from build123d import *

# Parameters (mm, degrees)
SKETCH063_W          = 88
SKETCH063_H          = 3
PAD030_DEPTH         = 176
SKETCH064_R          = 25
POCKET030_DEPTH      = 100
POCKET030_DEPTH_BACK = 100
PAD031_DEPTH         = 19
SKETCH066_W          = 139
SKETCH066_H          = 6
SKETCH066_W_2        = 6
SKETCH066_H_2        = 69.5
POCKET031_DEPTH      = 20
SKETCH067_W          = 3
SKETCH067_H          = 88
PAD032_DEPTH         = 19
SKETCH068_W          = 3
SKETCH068_H          = 79
PAD033_DEPTH         = 6
PAD033_DEPTH_BACK    = 6
CHAMFER009_SIZE      = 2.99
CHAMFER010_SIZE      = 1.5
FILLET017_R          = 2.99
SKETCH087_W          = 67
SKETCH087_H          = 4.5
PAD038_DEPTH         = 3
CHAMFER012_SIZE      = 2.99
CHAMFER014_SIZE      = 1


with BuildPart() as part:
    # Sketch063 → Pad030 (new body)
    with BuildSketch(Plane.YZ):
        with Locations((-44, 20.5)):
            Rectangle(SKETCH063_W, SKETCH063_H)
    extrude(amount=PAD030_DEPTH)

    # Sketch064 → Pocket030 (cut, two sides)
    with BuildSketch(Plane.XY) as pocket030_sk:
        with Locations((45.5, -45.5)):
            Circle(SKETCH064_R)
        with Locations((130.5, -45.5)):
            Circle(SKETCH064_R)
    extrude(amount=-POCKET030_DEPTH, mode=Mode.SUBTRACT)
    extrude(pocket030_sk.sketch, amount=POCKET030_DEPTH_BACK, mode=Mode.SUBTRACT)

    # Sketch065 → Pad031 (join)
    with BuildSketch(Plane.XY):
        with BuildLine():
            ThreePointArc((0, -12.5), (8.838835, -8.838835), (12.5, 0))
            Line((0, 0), (12.5, 0))
            Line((0, -12.5), (0, 0))
        make_face()
        with BuildLine():
            ThreePointArc((163.5, 0), (169.75, -6.25), (176, 0))
            Line((163.5, 0), (176, 0))
        make_face()
        with BuildLine():
            ThreePointArc((94.25, -88), (88, -81.75), (81.75, -88))
            Line((81.75, -88), (94.25, -88))
        make_face()
    extrude(amount=PAD031_DEPTH)

    # Sketch066 → Pocket031 (cut)
    with BuildSketch(Plane.XY):
        with Locations((88, -3)):
            Rectangle(SKETCH066_W, SKETCH066_H)
        with Locations((3, -53.25)):
            Rectangle(SKETCH066_W_2, SKETCH066_H_2)
    extrude(amount=POCKET031_DEPTH, mode=Mode.SUBTRACT)

    # Sketch067 → Pad032 (join)
    with BuildSketch(Plane.XY):
        with Locations((174.5, -44)):
            Rectangle(SKETCH067_W, SKETCH067_H)
    extrude(amount=PAD032_DEPTH)

    # Sketch068 → Pad033 (join, two sides)
    with BuildSketch(Plane.XY) as pad033_sk:
        with Locations((171.5, -48.5)):
            Rectangle(SKETCH068_W, SKETCH068_H)
    extrude(amount=PAD033_DEPTH)
    extrude(pad033_sk.sketch, amount=-PAD033_DEPTH_BACK)

    # Chamfer009
    chamfer009_edges = [part.edges().sort_by_distance(p)[0] for p in [
        (173, -48.5, 6),
    ]]
    chamfer(chamfer009_edges, length=CHAMFER009_SIZE)

    # Chamfer010
    chamfer010_edges = [part.edges().sort_by_distance(p)[0] for p in [
        (173, -48.5, -6),
    ]]
    chamfer(chamfer010_edges, length=CHAMFER010_SIZE)

    # Fillet017
    fillet017_edges = [part.edges().sort_by_distance(p)[0] for p in [
        (166.688138, -5.448624, 19),
        (88, -81.75, 19),
        (8.838835, -8.838835, 19),
    ]]
    fillet(fillet017_edges, radius=FILLET017_R)

    # Sketch087 → Pad038 (join)
    with BuildSketch(Plane.XY.offset(19)):
        with Locations((42.5, -87.25)):
            Rectangle(SKETCH087_W, SKETCH087_H)
        with Locations((133.5, -87.25)):
            Rectangle(SKETCH087_W, SKETCH087_H)
    extrude(amount=-PAD038_DEPTH)

    # Chamfer012
    chamfer012_edges = [part.edges().sort_by_distance(p)[0] for p in [
        (133.5, -85, 19),
        (42.5, -85, 19),
    ]]
    chamfer(chamfer012_edges, length=CHAMFER012_SIZE)

    # Chamfer014
    chamfer014_edges = [part.edges().sort_by_distance(p)[0] for p in [
        (88, -88, 0),
    ]]
    chamfer(chamfer014_edges, length=CHAMFER014_SIZE)


solid = part.part
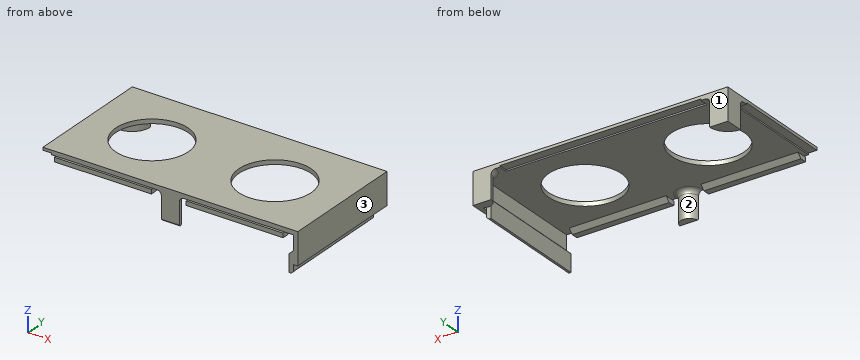
Could you check a few things on this model? Use its own coordinates, in mm. Face numbers are marked on the shaded views. Give positions to 0.01 mm unless a question says otherwise; leave off trailing zeros. Order: outer loops, then holes, each group sorted by start corner. A loop starts at its lowest first (then second) coordinate and runs counter-clockwise, first axis right, second up. Notation, with made-up numbers: M 63.5,1.5 L 114.5,1.5 A13 cw 114.5,17.5 Z; hole C -16.5,81.25 d2. An arc over 180 degrees is marked long. One line per question, with ' | ' between items.
1. If I drill on line 1 (X direction, y = -45.5, z = 20.2); line 2 (X direction, y = -45.5, z = 19.9); line 3 (Y direction, x = 45.5, z = 20.25), over which ranges is the centre line in solid material (lowest first)?
Results:
line 1: 0 to 20.5, 70.5 to 105.5, 155.5 to 176 | line 2: 6 to 20.5, 70.5 to 105.5, 155.5 to 176 | line 3: -88 to -70.5, -20.5 to 0
2. We'd pull the mould along X, two halves only. Please class the marked faces 1, 2 and 3: +X half, -X half, draft (parallel to the pull), parting line (faces both ways), or undercut.
Results:
face 1: draft | face 2: undercut | face 3: +X half
3. I want a section at C-C (y = -45.5). Give the number of separate pieces and of enclosed holes in the cut face, and give its area (3 significant figures).
Results:
separate pieces: 3 | enclosed holes: 0 | area: 318 mm²
4. I want a section at D-D (x = 88). List the corners of the cut face in (y, z) for me.
Results:
outline: M -88,1 L -87,0 L -81.75,0 L -81.75,16.01 A2.99 cw -78.76,19 L -6,19 L -6,20 L 0,20 L 0,22 L -88,22 Z
5. I want a section at A-A (z = 11). List the corners of the cut face in (x, y) for me, and give its area (3 significant figures).
Results:
outline: M 0,-12.5 A12.5 ccw 12.5,0 L 0,0 Z; M 81.75,-88 L 94.25,-88 A6.25 ccw Z; M 163.5,0 A6.25 ccw 173,-5.34 L 173,-88 L 176,-88 L 176,0 Z | area: 498 mm²
6. I'm going to push flat-ended pins straight in: pin 1 (4 mm diameter, centred on x = 26.5, y = -80.5, fed in from -Z); pin 2 (9.5 mm diameter, centred on y = -30, z = 2, fed in from -X); pin 3 (4 mm diameter, centred on x = 5, y = -7.5, fed in from -Z). Where does each tip first touch, or does it pass through?
Results:
pin 1: z = 18.51 | pin 2: x = 170 | pin 3: z = 0
